```python
from build123d import *

# Parameters (mm, degrees)
SKETCH_1_R          = 2.2
EXTRUDE_1_DEPTH     = 5
SKETCH_2_W          = 410
SKETCH_2_H          = 226.105378696
CUT_EXTRUDE_2_DEPTH = 5
SKETCH_4_W          = 410
SKETCH_4_H          = 19.486670542
EXTRUDE_3_DEPTH     = 5
SKETCH_5_R          = 3.3
CUT_EXTRUDE_3_DEPTH = 10


with BuildPart() as part:
    # 草图1 → 凸台-拉伸1 (new body)
    with BuildSketch(Plane.XY):
        Polygon((-200, 150), (200, 150), (200, 110), (205, 110), (205, 70), (200, 70), (200, 30), (205, 30), (205, -30), (200, -30), (200, -70), (205, -70), (205, -110), (200, -110), (200, -150), (160, -150), (160, -155), (120, -155), (120, -150), (80, -150), (80, -155), (40, -155), (40, -150), (-40, -150), (-40, -155), (-80, -155), (-80, -150), (-120, -150), (-120, -155), (-160, -155), (-160, -150), (-200, -150), (-200, -110), (-205, -110), (-205, -70), (-200, -70), (-200, -30), (-205, -30), (-205, 30), (-200, 30), (-200, 70), (-205, 70), (-205, 110), (-200, 110), align=None)
        with Locations((-140, -140)):
            Circle(SKETCH_1_R, mode=Mode.SUBTRACT)
        with Locations((-100, -140)):
            Circle(SKETCH_1_R, mode=Mode.SUBTRACT)
        with Locations((-60, -140)):
            Circle(SKETCH_1_R, mode=Mode.SUBTRACT)
        with Locations((-20, -140)):
            Circle(SKETCH_1_R, mode=Mode.SUBTRACT)
        with Locations((20, -140)):
            Circle(SKETCH_1_R, mode=Mode.SUBTRACT)
        with Locations((60, -140)):
            Circle(SKETCH_1_R, mode=Mode.SUBTRACT)
        with Locations((100, -140)):
            Circle(SKETCH_1_R, mode=Mode.SUBTRACT)
        with Locations((140, -140)):
            Circle(SKETCH_1_R, mode=Mode.SUBTRACT)
        with Locations((-190, 110)):
            Circle(SKETCH_1_R, mode=Mode.SUBTRACT)
        with Locations((-190, 70)):
            Circle(SKETCH_1_R, mode=Mode.SUBTRACT)
        with Locations((-190, 30)):
            Circle(SKETCH_1_R, mode=Mode.SUBTRACT)
        with Locations((-190, -30)):
            Circle(SKETCH_1_R, mode=Mode.SUBTRACT)
        with Locations((-190, -70)):
            Circle(SKETCH_1_R, mode=Mode.SUBTRACT)
        with Locations((-190, -110)):
            Circle(SKETCH_1_R, mode=Mode.SUBTRACT)
        with Locations((190, -110)):
            Circle(SKETCH_1_R, mode=Mode.SUBTRACT)
        with Locations((190, -70)):
            Circle(SKETCH_1_R, mode=Mode.SUBTRACT)
        with Locations((190, -30)):
            Circle(SKETCH_1_R, mode=Mode.SUBTRACT)
        with Locations((190, 30)):
            Circle(SKETCH_1_R, mode=Mode.SUBTRACT)
        with Locations((190, 70)):
            Circle(SKETCH_1_R, mode=Mode.SUBTRACT)
        with Locations((190, 110)):
            Circle(SKETCH_1_R, mode=Mode.SUBTRACT)
    extrude(amount=EXTRUDE_1_DEPTH)

    # 草图2 → 切除-拉伸2 (cut)
    with BuildSketch(Plane.XY.offset(5)):
        with Locations((0, 43.052689348)):
            Rectangle(SKETCH_2_W, SKETCH_2_H)
    extrude(amount=-CUT_EXTRUDE_2_DEPTH, mode=Mode.SUBTRACT)

    # 草图4 → 凸台-拉伸3 (add)
    with BuildSketch(Plane.XY.offset(5)):
        with Locations((0, -79.743335271)):
            Rectangle(SKETCH_4_W, SKETCH_4_H)
    extrude(amount=-EXTRUDE_3_DEPTH)

    # 草图5 → 切除-拉伸3 (cut)
    with BuildSketch(Plane(origin=(0, 0, 0), x_dir=(-1, 0, 0), z_dir=(0, 0, -1))):
        with Locations((-80, -89.5)):
            Circle(SKETCH_5_R)
        with Locations((-128, -89.5)):
            Circle(SKETCH_5_R)
        with Locations(Location((128, -89.5, 0), (0, 0, 180))):
            Circle(SKETCH_5_R)
        with Locations(Location((80, -89.5, 0), (0, 0, 180))):
            Circle(SKETCH_5_R)
    extrude(amount=-CUT_EXTRUDE_3_DEPTH, mode=Mode.SUBTRACT)


solid = part.part
```
CAD build for the part. Positions are in the model's coordinates, mm. Round coordinates to 2 decimals unless told otherwise and drop trailing zeros. Order: outer loops, then holes, each group sorted by start corner. A loop starts at its lowest first (then second) coordinate and runs counter-clockwise, first axis right, second up.
Item 1: Probe line 1 along Y through (x, z) = (-128, 2.6); line 2 along Y through (x, z) = (183, 4.1); line 3 along X through (y, z) = (-91.5, 1.7). List the from-to ranges inside material, lowest first.
Item 2: Mould opens along X. For faces 1 (the face through (130.43, -87.27, 2.46)), 2 (the face through (3, -112, 5)) say: pulls with the +X half, pulls with the -X half, needs draft (parallel to the pull), parting line crosses it, or undercut.
Item 3: Saw through at B-B on x = -177. Write the cut outline in (y, z), then the cut area to 3 significant figures.
Item 4: Saw through at A-A on z = 2.95. State how many separate pieces and enclosed holes the cut face has, then the cut area to 3 significant figures.
Item 5: Pin check, flat tips, straight feed: pin 1 (1.5 mm diameter, centred on x = -12.5, z = 1.5, fed in from -Y); pin 2 (3 mm diameter, centred on y = -112, z = 4, fed in from +X); pin 3 (1 mm diameter, centred on y = -119, z = 4, fed in from -X). Stop position of each tip, or through.
Reported:
1. line 1: y = -155 to -92.8, -86.2 to -70
1. line 2: y = -150 to -70
1. line 3: x = -205 to -130.62, -125.38 to -82.62, -77.38 to 77.38, 82.62 to 125.38, 130.62 to 205
2. face 1: undercut
2. face 2: needs draft
3. outline: (-150, 0) - (-70, 0) - (-70, 5) - (-150, 5) - close
3. area: 400 mm2
4. separate pieces: 1
4. enclosed holes: 14
4. area: 32,900 mm2
5. pin 1: stops at y = -150
5. pin 2: stops at x = 200
5. pin 3: stops at x = -200
